Check sheet for the modelled part. Datum: model origin and axes. Units: mm. Face numbers are marked on the shaded views. A direction names the side the tool comes from. Give positions to 0.01 mm unless a question says otherwise; leave off trailing zeros. Order: outer loops, then holes, each group sorted by start corner. A loop starts at its lowest first (then second) coordinate and runs counter-clockwise, first axis right, second up.
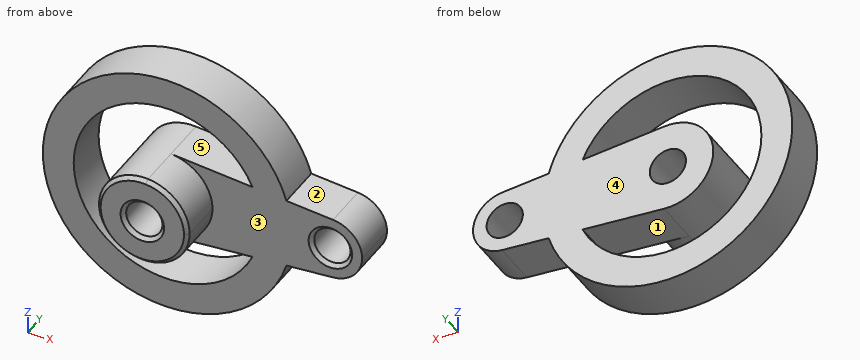
from build123d import *

# Parameters (mm, degrees)
F0_R     = 10
F1_DEPTH = 25
F2_DEPTH = 50
F3_SIZE  = 2
F4_R     = 68.61461
F4_R_2   = 51.589695
F5_DEPTH = 25


with BuildPart() as f1:
    # F0 (on Front) → F1 (new body)
    with BuildSketch(Plane.XZ):
        with BuildLine():
            ThreePointArc((2.083333, -24.913043), (18.399502, -16.92508), (25, 0))
            ThreePointArc((25, 0), (18.399502, 16.92508), (2.083333, 24.913043))
            ThreePointArc((2.083333, 24.913043), (-25, 0), (2.083333, -24.913043))
        make_face()
        Circle(F0_R, mode=Mode.SUBTRACT)
        with BuildLine():
            ThreePointArc((2.083333, 24.913043), (18.399502, 16.92508), (25, 0))
            ThreePointArc((25, 0), (18.399502, -16.92508), (2.083333, -24.913043))
            Line((2.083333, -24.913043), (91.458333, -17.43913))
            ThreePointArc((91.458333, -17.43913), (72.5, 0), (91.458333, 17.43913))
            Line((91.458333, 17.43913), (2.083333, 24.913043))
        make_face()
        with BuildLine():
            ThreePointArc((107.5, 0), (102.879651, 11.847556), (91.458333, 17.43913))
            ThreePointArc((91.458333, 17.43913), (72.5, 0), (91.458333, -17.43913))
            ThreePointArc((91.458333, -17.43913), (102.879651, -11.847556), (107.5, 0))
        make_face()
        with Locations((90, 0)):
            Circle(F0_R, mode=Mode.SUBTRACT)
    extrude(amount=F1_DEPTH)

    # F0 (on Front) → F2 (join)
    with BuildSketch(Plane.XZ):
        with BuildLine():
            ThreePointArc((2.083333, -24.913043), (18.399502, -16.92508), (25, 0))
            ThreePointArc((25, 0), (18.399502, 16.92508), (2.083333, 24.913043))
            ThreePointArc((2.083333, 24.913043), (-25, 0), (2.083333, -24.913043))
        make_face()
        Circle(F0_R, mode=Mode.SUBTRACT)
    extrude(amount=F2_DEPTH)

    # F3
    f3_edges = [f1.edges().sort_by_distance(p)[0] for p in [
        (-2.083333, -50, 24.913043),
        (-10, -50, 0),
        (80, -25, 0),
    ]]
    chamfer(f3_edges, length=F3_SIZE)

    # F4 (on Front) → F5 (join)
    with BuildSketch(Plane.XZ):
        Circle(F4_R)
        Circle(F4_R_2, mode=Mode.SUBTRACT)
    extrude(amount=F5_DEPTH)


solid = f1.part
1) Section check B-B, the plane z = 41.5. Record the cut outline in (x, y), then the cut area to 3 significant figures.
Recorded:
outline: (-54.64, -25) - (-30.65, -25) - (-30.65, 0) - (-54.64, 0) - close; (30.65, -25) - (54.64, -25) - (54.64, 0) - (30.65, 0) - close
area: 1,200 mm2
2) Draft check along X on the marked faces 1, 2 and 3. Enter one of: +X half, -X half, draft (parallel to the pull), parting line (faces both ways), or undercut.
Recorded:
face 1: undercut
face 2: +X half
face 3: draft
3) Section check A-A, the plane x = 0. Record the cut outline in (y, z).
Recorded:
outline: (-50, -23) - (-48, -25) - (0, -25) - (0, -10) - (-48, -10) - (-50, -12) - close; (-50, 12) - (-48, 10) - (0, 10) - (0, 25) - (-48, 25) - (-50, 23) - close; (-25, -68.61) - (0, -68.61) - (0, -51.59) - (-25, -51.59) - close; (-25, 51.59) - (0, 51.59) - (0, 68.61) - (-25, 68.61) - close
4) Set-up check for the marked faces 4 and 5: record each of +Z, -Z, +X, -X, +Y, -Y from which the full face is reachable in a straight line by a thin tool's end or side.
Recorded:
face 4: +Z, -Z, +X, -X, +Y
face 5: +Y, -Y
5) Section check C-C, the plane y = -21. Record the cut outline in (x, z).
Recorded:
outline: (65.76, -19.59) - (91.46, -17.44) arc R17.5 ccw to (91.46, 17.44) - (65.76, 19.59) arc R68.61 ccw (long way) to start; hole circle Ø20 at (0, 0); hole (2.08, -24.91) arc R25 cw (long way) to (2.08, 24.91) - (47.05, 21.15) arc R51.59 ccw (long way) to (47.05, -21.15) - close; hole circle Ø20 at (90, 0)
6) Material ranges on L1, parallel to Z at x = 0, y = -17; L2, parallel to Z at x = 0, y = -26; L3, parallel to Z at x = 23.5, y = -5.5, recorded low to high.
Recorded:
L1: z = -68.61 to -51.59, -25 to -10, 10 to 25, 51.59 to 68.61
L2: z = -25 to -10, 10 to 25
L3: z = -64.46 to -45.93, -23.12 to 23.12, 45.93 to 64.46
7) Depth check by flat-ended pin: pin 1 Ø8 at (x, z) = (49.5, 16) entering from -Y; pin 2 Ø16 at (x, z) = (0, 0) entering from -Y; pin 3 Ø4 at (y, z) = (-39, -7) entering from -X; pin 4 Ø5 at (y, z) = (-38, -5) entering from +X. Enter the tip coordinate at first touch or a pass-through.
Recorded:
pin 1: stops at y = -25
pin 2: passes through
pin 3: stops at x = -24.49
pin 4: stops at x = 24.87
8) Section check D-D, the plane x = 39. Record the cut outline in (y, z).
Recorded:
outline: (-25, -56.45) - (0, -56.45) - (0, -33.77) - (-25, -33.77) - close; (-25, -21.83) - (0, -21.83) - (0, 21.83) - (-25, 21.83) - close; (-25, 33.77) - (0, 33.77) - (0, 56.45) - (-25, 56.45) - close
